```python
from build123d import *

# Parameters (mm, degrees)
SKETCH1_R           = 6.35
BOSS_EXTRUDE1_DEPTH = 15.24


with BuildPart() as part:
    # Sketch1 → Boss-Extrude1 (new body)
    with BuildSketch(Plane(origin=(0, 0, 0), x_dir=(1, 0, 0), z_dir=(0, 1, 0))):
        Polygon((0, 0), (0, -38.1), (38.1, -63.5), (101.6, -63.5), (127, -38.1), (127, 0), (101.6, 0), (79.248, -22.352), (47.752, -22.352), (25.4, 0), align=None)
        with Locations((19.05, -19.05)):
            Circle(SKETCH1_R, mode=Mode.SUBTRACT)
        with Locations((44.45, -38.1)):
            Circle(SKETCH1_R, mode=Mode.SUBTRACT)
        with Locations((91.948, -41.148)):
            Circle(SKETCH1_R, mode=Mode.SUBTRACT)
        with Locations((111.252, -25.4)):
            Circle(SKETCH1_R, mode=Mode.SUBTRACT)
    extrude(amount=BOSS_EXTRUDE1_DEPTH)


solid = part.part
```
Can you work these out from the model? Positions are in its coordinate system, mm. A direction names the side the tool comes from. Coordinates: 2 decimals unless noted, no trailing zeros. Loops run counter-clockwise (first coordinate to the right, second up) from the corner with the lowest first, then second, coordinate; pieces in that order, holes last. Notation, with made-up numbers: (-5, 57) -> (26, 57) arc R21 ccw to (26, 80) -> close; hole circle Ø9 at (-15.75, -0.5). An arc over 180 degrees is marked (long way). Put each result on its own line as item: value. Start each with the question number.
Q1. If I drill on line 1 (X direction, y = 2.5, z = 17); line 2 (X direction, y = 1, z = 14); line 3 (X direction, y = 5, z = 45), over which ranges is the centre line in solid material (lowest first)? Write a range as [from, to].
Q2. I want a section at A-A (x = 19.05). Write out the boundary of the cut face in (y, z).
Q3. I want a section at B-B (z = 15.5). Write out the boundary of the cut face in (x, y), plus the area to 3 significant figures.
Q4. For faces 4 (the face through (64, 8, 22.352)), 5 (the face through (63, 0, 31)), which set-ups out of +Z, -Z, +X, -X, +Y, -Y let a thin tool reach every point of the face, with its end or its side?
Q5. I want a section at C-C (y = 12.75). Write out the boundary of the cut face in (x, z).
Q6. I'm going to push flat-ended pins straight in: P1, Ø1, axis at x = 50, z = 50.5, coming from the -Y side; P2, Ø11.5, axis at x = 44.45, z = 38.1, coming from the +Y side. Where does each tip first touch, or does it pass through?
Q7. I want a section at D-D (x = 44.45). Write out the boundary of the cut face in (y, z).
Q8. Thinking about a two-plate mould opening in Z: for faces 1 (the face through (114, 8, 0)), 2 (the face through (24.916, 7.513, 21.482)), 3 (the face through (114.1, 7.5, 51)), which applies, pulls with the +Z half, pulls with the -Z half, needs draft (parallel to the pull), parting line crosses it, or undercut?
Taken from the geometry:
1. line 1: x = [0, 13.04], [25.06, 42.4], [84.6, 127]
1. line 2: x = [0, 15.2], [22.9, 39.4], [87.6, 127]
1. line 3: x = [10.35, 86.9], [97, 120.1]
2. outline: (0, 0) -> (15.24, 0) -> (15.24, 12.7) -> (0, 12.7) -> close; (0, 25.4) -> (15.24, 25.4) -> (15.24, 50.8) -> (0, 50.8) -> close
3. outline: (0, 0) -> (13.79, 0) -> (13.79, 15.24) -> (0, 15.24) -> close; (24.31, 0) -> (40.9, 0) -> (40.9, 15.24) -> (24.31, 15.24) -> close; (86.1, 0) -> (127, 0) -> (127, 15.24) -> (86.1, 15.24) -> close
3. area: 1,090 mm2
4. face 4: -Z, +Y, -Y
4. face 5: +Z, -Z, +X, -X, -Y
5. outline: (0, 0) -> (25.4, 0) -> (47.75, 22.35) -> (79.25, 22.35) -> (101.6, 0) -> (127, 0) -> (127, 38.1) -> (101.6, 63.5) -> (38.1, 63.5) -> (0, 38.1) -> close; hole circle Ø12.7 at (19.05, 19.05); hole circle Ø12.7 at (44.45, 38.1); hole circle Ø12.7 at (91.95, 41.15); hole circle Ø12.7 at (111.25, 25.4)
6. P1: stops at y = 0
6. P2: passes through
7. outline: (0, 19.05) -> (15.24, 19.05) -> (15.24, 31.75) -> (0, 31.75) -> close; (0, 44.45) -> (15.24, 44.45) -> (15.24, 63.5) -> (0, 63.5) -> close
8. face 1: pulls with the -Z half
8. face 2: undercut
8. face 3: pulls with the +Z half
